```python
from build123d import *

# Parameters (mm, degrees)
F0_R      = 14
F0_R_2    = 11
F1_DEPTH  = 6
F2_W      = 57
F2_H      = 57
F3_DEPTH  = 6
F5_W      = 3
F5_H      = 50.979116
F5_H_2    = 51
F6_DEPTH  = 1
F7_W      = 6
F7_H      = 50.96702
F7_W_2    = 3
F7_H_2    = 50.979116
F8_DEPTH  = 1
F9_W      = 6.5
F9_H      = 57
F9_R      = 2
F10_DEPTH = 6


with BuildPart() as f1:
    # F0 (on Top) → F1 (new body)
    with BuildSketch(Plane.XY):
        Circle(F0_R)
        Circle(F0_R_2, mode=Mode.SUBTRACT)
    extrude(amount=F1_DEPTH)


with BuildPart() as f3:
    # F2 (on face) → F3 (new body)
    with BuildSketch(Plane(origin=(0, 0, 0), x_dir=(1, 0, 0), z_dir=(0, 0, -1))):
        Rectangle(F2_W, F2_H)
        Polygon((25.5, -2.533051), (25.5, -25.5), (2.32699, -25.5), (-2.32699, -25.5), (-25.5, -25.5), (-25.5, -2.533051), (-25.5, 2.533051), (-25.5, 25.5), (-2.32699, 25.5), (2.32699, 25.5), (25.5, 25.5), (25.5, 2.533051), align=None, mode=Mode.SUBTRACT)
        with BuildLine():
            Line((2.32699, 13.805257), (2.32699, 25.5))
            Line((2.32699, 25.5), (-2.32699, 25.5))
            Line((-2.32699, 25.5), (-2.32699, 13.805257))
            ThreePointArc((-2.32699, 13.805257), (0, 14), (2.32699, 13.805257))
        make_face()
        with BuildLine():
            Line((-25.5, 2.533051), (-25.5, -2.533051))
            Line((-25.5, -2.533051), (-13.768938, -2.533051))
            ThreePointArc((-13.768938, -2.533051), (-14, 0), (-13.768938, 2.533051))
            Line((-13.768938, 2.533051), (-25.5, 2.533051))
        make_face()
        with BuildLine():
            Line((-2.32699, -25.5), (2.32699, -25.5))
            Line((2.32699, -25.5), (2.32699, -13.805257))
            ThreePointArc((2.32699, -13.805257), (0, -14), (-2.32699, -13.805257))
            Line((-2.32699, -13.805257), (-2.32699, -25.5))
        make_face()
        with BuildLine():
            Line((13.768938, -2.533051), (25.5, -2.533051))
            Line((25.5, -2.533051), (25.5, 2.533051))
            Line((25.5, 2.533051), (13.768938, 2.533051))
            ThreePointArc((13.768938, 2.533051), (13.942115, 1.271784), (14, 0))
            ThreePointArc((14, 0), (13.942115, -1.271784), (13.768938, -2.533051))
        make_face()
    extrude(amount=-F3_DEPTH)


with BuildPart() as f1_1:
    add(f1.part)

    # F4: union F3
    add(f3.part)

    # F5 (on face) → F6 (join)
    with BuildSketch(Plane(origin=(0, 0, 0), x_dir=(1, 0, 0), z_dir=(0, 0, -1))):
        with Locations((27, -0.010442)):
            Rectangle(F5_W, F5_H)
        with Locations((-27, 0)):
            Rectangle(F5_W, F5_H_2)
    extrude(amount=F6_DEPTH)

    # F7 (on face) → F8 (join)
    with BuildSketch(Plane(origin=(0, 0, -1), x_dir=(1, 0, 0), z_dir=(0, 0, -1))):
        with Locations((-25.5, -0.004394)):
            Rectangle(F7_W, F7_H)
        with Locations((24, -0.010442)):
            Rectangle(F7_W_2, F7_H_2)
        with Locations((27, -0.010442)):
            Rectangle(F7_W_2, F7_H_2)
    extrude(amount=F8_DEPTH)

    # F9 (on Top) → F10 (join)
    with BuildSketch(Plane.XY):
        with Locations((-31.75, 0)):
            Rectangle(F9_W, F9_H)
        with Locations((-32, -23.5)):
            Circle(F9_R, mode=Mode.SUBTRACT)
        with Locations((-32, 23.5)):
            Circle(F9_R, mode=Mode.SUBTRACT)
        with Locations((31.75, 0)):
            Rectangle(F9_W, F9_H)
        with Locations((32, -23.5)):
            Circle(F9_R, mode=Mode.SUBTRACT)
        with Locations((32, 23.5)):
            Circle(F9_R, mode=Mode.SUBTRACT)
    extrude(amount=F10_DEPTH)


solid = f1_1.part
```
Can you work these out from the model? Positions are in its coordinate system, mm. A direction names the side the tool comes from. Give positions to 0.01 mm unless a question says otherwise; leave off trailing zeros. Order: outer loops, then holes, each group sorted by start corner. A loop starts at its lowest first (then second) coordinate and runs counter-clockwise, first axis right, second up. Notation, with made-up numbers: M -12.5,25 L 14.5,25 A16 ccw 14.5,34 Z; hole C -16.5,67.5 d8. An arc over 180 degrees is marked long. Write item = value, one per line. Start each with the question number.
Q1. We'd pull the mould along Y, two halves only. Please class faces 1 (the flat face through (26, -25.479, -1)), 2 (the flat face through (2.327, -20, 3)), 3 (the flat face through (26, 25.5, -1)): pulls with the +Y half, pulls with the -Y half, needs draft (parallel to the pull), parting line crosses it, or undercut.
Q2. For faces 4 (the flat face through (20, -2.533, 3)), 5 (the cylindrical face through (-9.9, -9.9, 3)), 6 (the flat face through (28.5, 0, -1)), which set-ups out of +Z, -Z, +X, -X, +Y, -Y let a thin tool reach every point of the face, with its end or its side?
Q3. I need wall thicknesses on probe 1 along X at (y, z) = (-15, 2.75); probe 2 along Y at (x, z) = (-32, 3.7); probe 3 along X at (y, z) = (4, -0.25). Which ranges of each line are inside material? Lowest first, please. Write a range as [from, to].
Q4. Suppose I cut it at D-D (x = 0). Write out the boundary of the cut face in (y, z).
Q5. Will these pins go through, and if not, where does the flat tip stop? pin 1 Ø5 at (x, y) = (-1, -9) entering from -Z; pin 2 Ø6 at (x, y) = (-6.5, 20) entering from +Z; pin 3 Ø0.8 at (x, z) = (-26.5, -0.5) entering from +Y; pin 4 Ø1 at (y, z) = (0.5, -1) entering from -X.
Q6. Suppose I cut it at A-A (y = 0). Write out the boundary of the cut face in (x, z).
Q7. Suppose I cut it at C-C (z = 3.5). Count the separate pieces of the cut face and the enclosed holes in it, plus the area to 3 significant figures.
Q8. Suppose I cut it at B-B (x = 32). Write out the boundary of the cut face in (y, z).
Check result:
q1.face_1 = pulls with the -Y half
q1.face_2 = undercut
q1.face_3 = pulls with the +Y half
q2.face_4 = +Z
q2.face_5 = +Z, -Z
q2.face_6 = -Z, +X, +Y, -Y
q3.probe_1 = [-35, -25.5], [-2.33, 2.33], [25.5, 35]
q3.probe_2 = [-28.5, -25.5], [-21.5, 21.5], [25.5, 28.5]
q3.probe_3 = [-28.5, -25.5], [25.5, 28.5]
q4.outline = M -28.5,0 L -11,0 L -11,6 L -28.5,6 Z; M 11,0 L 28.5,0 L 28.5,6 L 11,6 Z
q5.pin_1 = 0
q5.pin_2 = through
q5.pin_3 = 25.5
q5.pin_4 = -28.5
q6.outline = M -35,0 L -28.5,0 L -28.5,-2 L -22.5,-2 L -22.5,-1 L -25.5,-1 L -25.5,0 L -11,0 L -11,6 L -35,6 Z; M 11,0 L 25.5,0 L 25.5,-1 L 22.5,-1 L 22.5,-2 L 28.5,-2 L 28.5,0 L 35,0 L 35,6 L 11,6 Z
q7.separate_pieces = 1
q7.enclosed_holes = 9
q7.area = 1,800 mm2
q8.outline = M -28.5,0 L -25.5,0 L -25.5,6 L -28.5,6 Z; M -21.5,0 L 21.5,0 L 21.5,6 L -21.5,6 Z; M 25.5,0 L 28.5,0 L 28.5,6 L 25.5,6 Z
